Job drawing, mm, ordinate dimensions from the low corner. One solid piece. A direction names the side the tool comes from. Give positions to 0.01 mm unless a question says otherwise; leave off trailing zeros. Order: outer loops, then holes, each group sorted by start corner. A loop starts at its lowest first (then second) coordinate and runs counter-clockwise, first axis right, second up. Notation, with made-up numbers: (-1, -2) -> (43, -2) arc R22 ccw to (43, 7) -> close; hole circle Ø3 at (9.25, 54). An arc over 180 degrees is marked (long way). Write item = value, one per line. Start each with the question number.
(1) Saw through at D-D, the plane y = 1. List the corners of the cut face in (x, z), then the cut area to 3 significant figures.
(2) Saw through at A-A, the plane y = 5.5. List the corners of the cut face in (x, z).
(3) Flat gauge pin, fed straight in: pin 1 (2.5 mm diameter, centred on x = 2, y = 10, fed in from +Z). Where does the tip first touch, or does it go through?
(4) Which spindle directions (+Z, -Z, +X, -X, +Y, -Y) get a long thin tool onto all of the face, cutting with end or side? Do the marked faces 5 and 6. Say none if no direction does.
(5) Saw through at B-B, the plane z = 3. List the corners of the cut face in (x, y), then the cut area to 3 significant figures.
(6) Probe line 1 along Y through (x, z) = (28, 3.55); line 2 along X through (y, z) = (10, 2.1); line 3 along Y through (x, z) = (12.25, 2.7). List the from-to ranges inside material, lowest first. Write a range as from..to.
(7) Two-plate mould, pull along Y, no slides. Class the marked faces 1, 2, 3 and 4: pulls with the +Y half, pulls with the -Y half, needs draft (parallel to the pull), parting line crosses it, or undercut.
(8) Saw through at C-C, the plane x = 9.5. List the corners of the cut face in (y, z), then the cut area to 3 significant figures.
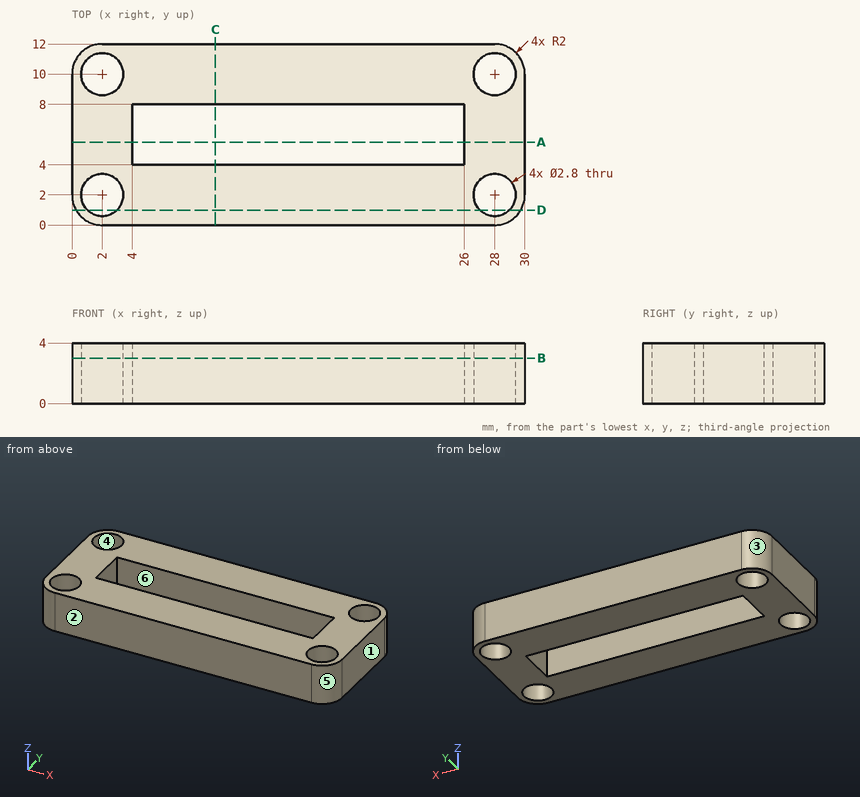
Results list:
q1.outline = (0.27, 0) -> (1.02, 0) -> (1.02, 4) -> (0.27, 4) -> close; (2.98, 0) -> (27.02, 0) -> (27.02, 4) -> (2.98, 4) -> close; (28.98, 0) -> (29.73, 0) -> (29.73, 4) -> (28.98, 4) -> close
q1.area = 102 mm^2
q2.outline = (0, 0) -> (4, 0) -> (4, 4) -> (0, 4) -> close; (26, 0) -> (30, 0) -> (30, 4) -> (26, 4) -> close
q3.pin_1 = through
q4.face_5 = +Z, -Z, +X, -Y
q4.face_6 = +Z, -Z
q5.outline = (0, 2) arc R2 ccw to (2, 0) -> (28, 0) arc R2 ccw to (30, 2) -> (30, 10) arc R2 ccw to (28, 12) -> (2, 12) arc R2 ccw to (0, 10) -> close; hole circle Ø2.8 at (2, 2); hole circle Ø2.8 at (2, 10); hole (4, 4) -> (26, 4) -> (26, 8) -> (4, 8) -> close; hole circle Ø2.8 at (28, 2); hole circle Ø2.8 at (28, 10)
q5.area = 244 mm^2
q6.line_1 = 0..0.6, 3.4..8.6, 11.4..12
q6.line_2 = 0..0.6, 3.4..26.6, 29.4..30
q6.line_3 = 0..4, 8..12
q7.face_1 = needs draft
q7.face_2 = pulls with the -Y half
q7.face_3 = pulls with the +Y half
q7.face_4 = undercut
q8.outline = (0, 0) -> (4, 0) -> (4, 4) -> (0, 4) -> close; (8, 0) -> (12, 0) -> (12, 4) -> (8, 4) -> close
q8.area = 32.0 mm^2
